Work out the finished part from the listing and answer in its coordinate system (mm). Face numbers are marked on the shaded views. A direction names the side the tool comes from. Round coordinates to 2 decimals unless told otherwise and drop trailing zeros. Write each loop counter-clockwise with the first axis right and the second up, starting at its lowest first coordinate (ties: lowest second). Pieces come first, ordered by that corner, then holes. Notation, with made-up numbers: M 64.5,38 L 100.5,38 A23 cw 100.5,60 Z; hole C 22.5,29 d10. An arc over 180 degrees is marked long. One line per item, written item: value. Start each with the question number.
Q1. Find section C-C (x = 44.5). Write down the section's boundary in (y, z).
Q2. Find section A-A (y = 54). Write down the section's boundary in (x, z), and give its area (3 significant figures).
Q3. Find section B-B (z = -11.5). Write down the section's boundary in (x, y).
Q4. Given pin 1 Ø5 at (x, z) = (-46, 13.5) entering from +Y; pin 2 Ø4.5 at (x, z) = (111.125, -50.8) entering from +Y; pin 3 Ø4 at (x, z) = (-50.8, 111.125) entering from +Y, each flat-ended and moving along its own axis, determine where each tip first touches the part or whether it passes through.
Q5. A tool of negligible diameter and unlimited length cuts with its end or side. For the marked faces 1 and 2, from which of +Z, -Z, +X, -X, +Y, -Y can it reach the whole face along a straight path? Write none if from no direction.
Q6. Consider probe 1 along Z at (x, y) = (76.2, 170.75); probe 2 along X at (y, z) = (47.5, 15). Determine where each line is inside the solid, lowest interval first.
from build123d import *

# Parameters (mm, degrees)
SKETCH1_W                   = 241.3
SKETCH1_H                   = 241.3
SKETCH1_W_2                 = 203.2
SKETCH1_H_2                 = 203.2
EXTRUDE_THIN1_DEPTH         = 177.8
SKETCH2_W                   = 241.3
SKETCH2_H                   = 241.3
BOSS_EXTRUDE1_DEPTH         = 19.05
F_1_4_20_TAPPED_HOLE1_D     = 5.1054
F_1_4_20_TAPPED_HOLE1_DEPTH = 16.51
F_1_4_20_TAPPED_HOLE1_TIP   = 1.533816902


with BuildPart() as part:
    # Sketch1 → Extrude-Thin1 (new body)
    with BuildSketch(Plane(origin=(0, 0, 0), x_dir=(1, 0, 0), z_dir=(0, 1, 0))):
        Rectangle(SKETCH1_W, SKETCH1_H)
        Rectangle(SKETCH1_W_2, SKETCH1_H_2, mode=Mode.SUBTRACT)
    extrude(amount=EXTRUDE_THIN1_DEPTH)

    # Sketch2 → Boss-Extrude1 (add)
    with BuildSketch(Plane(origin=(0, 0, 0), x_dir=(1, 0, 0), z_dir=(0, 1, 0))):
        Rectangle(SKETCH2_W, SKETCH2_H)
    extrude(amount=-BOSS_EXTRUDE1_DEPTH)

    # 1/4-20 Tapped Hole1
    with Locations(Plane(origin=(0, 177.8, 0), x_dir=(1, 0, 0), z_dir=(0, 1, 0))):
        with Locations((-76.2, -111.125), (-111.125, 76.2), (-111.125, 50.8), (-111.125, 25.4), (-111.125, 0), (-111.125, -25.4), (-111.125, -50.8), (-111.125, -76.2), (111.125, -76.2), (111.125, -50.8), (111.125, -25.4), (111.125, 0), (111.125, 25.4), (111.125, 50.8), (111.125, 76.2), (-76.2, 111.125), (-50.8, 111.125), (-25.4, 111.125), (0, 111.125), (25.4, 111.125), (50.8, 111.125), (76.2, 111.125), (76.2, -111.125), (50.8, -111.125), (25.4, -111.125), (0, -111.125), (-25.4, -111.125), (-50.8, -111.125)):
            Hole(F_1_4_20_TAPPED_HOLE1_D / 2, depth=F_1_4_20_TAPPED_HOLE1_DEPTH)
            with Locations((0, 0, -(F_1_4_20_TAPPED_HOLE1_DEPTH + F_1_4_20_TAPPED_HOLE1_TIP / 2))):  # 118° drill point
                Cone(0, F_1_4_20_TAPPED_HOLE1_D / 2, F_1_4_20_TAPPED_HOLE1_TIP, mode=Mode.SUBTRACT)


solid = part.part
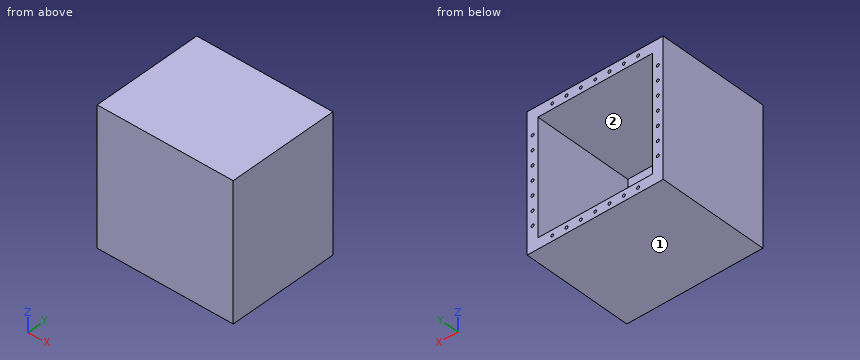
The answers:
1. outline: M -19.05,-120.65 L 177.8,-120.65 L 177.8,-101.6 L 0,-101.6 L 0,101.6 L 177.8,101.6 L 177.8,120.65 L -19.05,120.65 Z
2. outline: M -120.65,-120.65 L 120.65,-120.65 L 120.65,120.65 L -120.65,120.65 Z; hole M -101.6,-101.6 L 101.6,-101.6 L 101.6,101.6 L -101.6,101.6 Z
2. area: 16,900 mm2
3. outline: M -120.65,-19.05 L 120.65,-19.05 L 120.65,177.8 L 101.6,177.8 L 101.6,0 L -101.6,0 L -101.6,177.8 L -120.65,177.8 Z
4. pin 1: y = 0
4. pin 2: y = 161.11
4. pin 3: y = 160.96
5. face 1: -Z, +X, -X, +Y, -Y
5. face 2: +Y
6. probe 1: -120.65 to -113.68, -108.57 to -101.6, 101.6 to 108.57, 113.68 to 120.65
6. probe 2: -120.65 to -101.6, 101.6 to 120.65
